Read the model definition and answer for the solid it produces. Units are mm, in the model's axes. Face numbers are marked on the shaded views. A direction names the side the tool comes from. Give positions to 0.01 mm unless a question says otherwise; leave off trailing zeros. Order: outer loops, then holes, each group sorted by start corner. A loop starts at its lowest first (then second) coordinate and runs counter-clockwise, first axis right, second up. Notation, with made-up numbers: (74.5, -22) - (88.5, -22) arc R13 ccw to (88.5, -6) - close; hole circle Ø6 at (-35.75, -14.5). An arc over 180 degrees is marked (long way). Write each question's results on one line, items separated by ' | '.
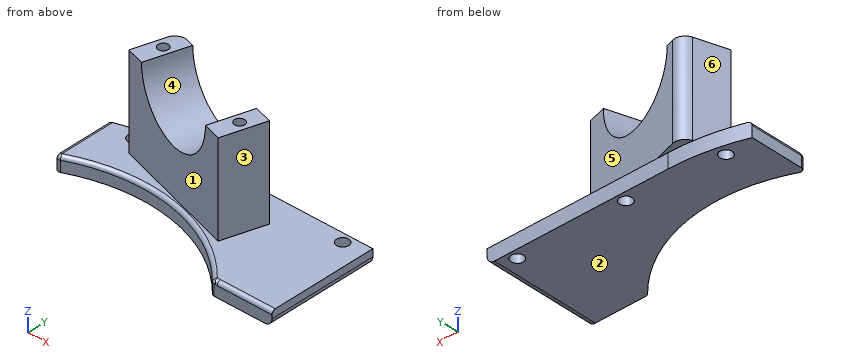
from build123d import *

# Parameters (mm, degrees)
PAD_DEPTH       = 4
PAD001_DEPTH    = 25.5
SKETCH002_R     = 12.9
POCKET_DEPTH    = 35.4050611872
FILLET_R        = 2
FILLET001_R     = 1
FILLET002_R     = 1
FILLET003_R     = 1
FILLET004_R     = 3
SKETCH003_R     = 1.4
POCKET001_DEPTH = 15
SKETCH004_R     = 1.7
POCKET002_DEPTH = 5


with BuildPart() as part:
    # Sketch → Pad (new body)
    with BuildSketch(Plane.XY):
        with BuildLine():
            Line((33.5410196625, 30), (50, 30))
            Line((50, 30), (50, 60))
            Line((0, 60), (50, 60))
            ThreePointArc((0, 60), (-10.1461187235, 59.1359135792), (-20, 56.5685424949))
            Line((-20, 40.3112887415), (-20, 56.5685424949))
            ThreePointArc((33.5410196625, 30), (8.5100218715, 44.1880020792), (-20, 40.3112887415))
        make_face()
    extrude(amount=PAD_DEPTH)

    # Sketch001 → Pad001 (new body)
    with BuildSketch(Plane.XY.offset(4)):
        Polygon((-5.671183324, 62.6409760428), (28.7557878907, 52.1155946728), (25.247327434, 40.6399376012), (-9.1796437807, 51.1653189712), align=None)
    extrude(amount=PAD001_DEPTH)

    # Sketch002 → Pocket (cut, through all)
    with BuildSketch(Plane(origin=(17.029415001, 55.7007066474, 0), x_dir=(-0.956304756, 0.2923717047, 0), z_dir=(0.2923717047, 0.956304756, 0))):
        with Locations((5.7378285358, 29.5)):
            Circle(SKETCH002_R)
    extrude(amount=-POCKET_DEPTH, mode=Mode.SUBTRACT)

    # Fillet
    fillet_edges = [part.edges().sort_by_distance(p)[0] for p in [
        (50, 45, 0),
    ]]
    fillet(fillet_edges, radius=FILLET_R)

    # Fillet001
    fillet001_edges = [part.edges().sort_by_distance(p)[0] for p in [
        (-20, 48.439916, 4),
    ]]
    fillet(fillet001_edges, radius=FILLET001_R)

    # Fillet002
    fillet002_edges = [part.edges().sort_by_distance(p)[0] for p in [
        (9.054169, 44.079724, 4),
    ]]
    fillet(fillet002_edges, radius=FILLET002_R)

    # Fillet003
    fillet003_edges = [part.edges().sort_by_distance(p)[0] for p in [
        (42.435596, 30, 4),
    ]]
    fillet(fillet003_edges, radius=FILLET003_R)

    # Fillet004
    fillet004_edges = [part.edges().sort_by_distance(p)[0] for p in [
        (-5.671183, 62.640976, 16.75),
    ]]
    fillet(fillet004_edges, radius=FILLET004_R)

    # Sketch003 → Pocket001 (cut)
    with BuildSketch(Plane.XY.offset(29.5)):
        with Locations((-4.7794903371, 56.6647829722)):
            Circle(SKETCH003_R)
        with Locations((24.6746961465, 47.6597344667)):
            Circle(SKETCH003_R)
    extrude(amount=-POCKET001_DEPTH, mode=Mode.SUBTRACT)

    # Sketch004 → Pocket002 (cut)
    with BuildSketch(Plane.XY.offset(4)):
        with Locations((44, 57.5)):
            Circle(SKETCH004_R)
        with Locations((-12, 55.75)):
            Circle(SKETCH004_R)
        with Locations((14, 57.5)):
            Circle(SKETCH004_R)
    extrude(amount=-POCKET002_DEPTH, mode=Mode.SUBTRACT)


solid = part.part
(1) Each of these flat-tipped pins is pushed along its axis until it touches: pin 1 (1.4 mm diameter, centred on x = 24.5, y = 47.5, fed in from +Z); pin 2 (3 mm diameter, centred on x = 18.5, z = 4.5, fed in from -Y); pin 3 (10 mm diameter, centred on x = 4, y = 38.5, fed in from -Z); pin 4 (1.5 mm diameter, centred on x = 24, z = 6.5, fed in from +Y). Where does it stop, or does it pass through?
Conclusion:
pin 1: z = 14.5 | pin 2: y = 40.64 | pin 3: through | pin 4: y = 53.8
(2) Section A-A (x = 44) is taken. Give the vertices of the cut face in (y, z), plus the area to 3 significant figures.
Conclusion:
outline: (30, 0) - (55.8, 0) - (55.8, 4) - (31, 4) arc R1 ccw to (30, 3) - close; (59.2, 0) - (60, 0) - (60, 4) - (59.2, 4) - close | area: 106 mm^2
(3) Section B-B (z = 18.75) is taken. Give the vertices of the cut face in (x, y).
Conclusion:
outline: (-9.18, 51.17) - (1.21, 47.99) - (4.72, 59.46) - (-2.8, 61.76) arc R3 ccw to (-6.55, 59.77) - close; (14.85, 43.82) - (25.25, 40.64) - (28.76, 52.12) - (18.36, 55.29) - close; hole circle Ø2.8 at (-4.78, 56.66); hole circle Ø2.8 at (24.67, 47.66)
(4) Consider probe 1 along Z at (x, y) = (31, 55); probe 2 along Y at (x, z) = (-5, 27.25); probe 3 along Y at (x, z) = (-12, 2.55). Determine where each line is inside the solid, lowest interval first. Write a range as [from, to].
Conclusion:
probe 1: [0, 4] | probe 2: [49.89, 55.28], [58.05, 61.59] | probe 3: [43.37, 54.05], [57.45, 58.79]
(5) The mould has two halves that part along X. Classify the marked faces 4, 5 and 6: pulls with the +X half, pulls with the -X half, needs draft (parallel to the pull), parting line crosses it, or undercut.
Conclusion:
face 4: undercut | face 5: pulls with the +X half | face 6: pulls with the -X half
(6) Section C-C (z = 9.25) is taken. Give the vertices of the cut face in (x, y).
Conclusion:
outline: (-9.18, 51.17) - (25.25, 40.64) - (28.76, 52.12) - (-2.8, 61.76) arc R3 ccw to (-6.55, 59.77) - close
(7) For the marked faces 1, 2 and 3, determine the directions among +Z, -Z, +X, -X, +Y, -Y from which every point of the face is accessible in a straight line to the end or side of a thin tool.
Conclusion:
face 1: +Z, -X, -Y | face 2: -Z, +X, -X, +Y, -Y | face 3: +Z, +X, -Y
